from build123d import *

# Parameters (mm, degrees)
BOSS_EXTRUDE1_DEPTH = 5
CIRPATTERN1_COUNT   = 3
CIRPATTERN1_ANGLE   = 120
SKETCH8_R           = 22.5
BOSS_EXTRUDE4_DEPTH = 10
SKETCH11_R          = 22.5
CUT_EXTRUDE4_DEPTH  = 11.7
SKETCH12_R          = 4
CUT_EXTRUDE5_DEPTH  = 3.3
SKETCH14_R          = 3.65
CUT_EXTRUDE7_DEPTH  = 100.784323589
CIRPATTERN2_COUNT   = 6
CUT_EXTRUDE9_DEPTH  = 15


# Read off the part's stored shape, not the designer's step: Boundary2
with BuildPart() as part:
    # Sketch1 → Boss-Extrude1 (new body)
    with BuildSketch(Plane(origin=(0, 0, 0), x_dir=(1, 0, 0), z_dir=(0, 1, 0))):
        with BuildLine():
            ThreePointArc((-15.9, 47.404535648), (-50, 0), (-15.9, -47.404535648))
            Line((-15.9, -47.404535648), (-15.9, 47.404535648))
        make_face()
        with BuildLine():
            ThreePointArc((-15.9, -47.404535648), (0, -50), (15.9, -47.404535648))
            Line((15.9, -47.404535648), (15.9, 47.404535648))
            ThreePointArc((15.9, 47.404535648), (0, 50), (-15.9, 47.404535648))
            Line((-15.9, 47.404535648), (-15.9, -47.404535648))
        make_face()
        with BuildLine():
            Line((-15.9, -70.5), (15.9, -70.5))
            Line((15.9, -70.5), (15.9, -47.404535648))
            ThreePointArc((15.9, -47.404535648), (0, -50), (-15.9, -47.404535648))
            Line((-15.9, -47.404535648), (-15.9, -70.5))
        make_face()
        with BuildLine():
            ThreePointArc((-15.9, 47.404535648), (0, 50), (15.9, 47.404535648))
            Line((15.9, 47.404535648), (15.9, 70.5))
            Line((15.9, 70.5), (-15.9, 70.5))
            Line((-15.9, 70.5), (-15.9, 47.404535648))
        make_face()
        with BuildLine():
            Line((15.9, 47.404535648), (15.9, -47.404535648))
            ThreePointArc((15.9, -47.404535648), (40.589407485, -29.197602641), (50, 0))
            ThreePointArc((50, 0), (40.589407485, 29.197602641), (15.9, 47.404535648))
        make_face()
    boss_extrude1 = extrude(amount=BOSS_EXTRUDE1_DEPTH)

    # CirPattern1: Boss-Extrude1 ×3 about axis
    cirpattern1_axis = Axis((0, 0, 0), (0, 1, 0))
    for i in range(1, CIRPATTERN1_COUNT):
        add(boss_extrude1.rotate(cirpattern1_axis, i * CIRPATTERN1_ANGLE / (CIRPATTERN1_COUNT - 1)))

    # Sketch8 → Boss-Extrude4 (add)
    with BuildSketch(Plane(origin=(0, 5, 0), x_dir=(1, 0, 0), z_dir=(0, 1, 0))):
        with Locations(Location((0, 0, 0), (0, 0, 270))):
            Circle(SKETCH8_R)
    extrude(amount=BOSS_EXTRUDE4_DEPTH)

    # Boundary2 outline → Boundary2 (revolve)
    with BuildSketch(Plane.XY):
        Polygon((32.5, 5), (22.499998072, 15.000001928), (22.5, 5), align=None)
    revolve(axis=Axis((0, 0, 0), (0, 1, 0)))

    # Sketch11 → Cut-Extrude4 (cut)
    with BuildSketch(Plane.XZ):
        with Locations(Location((0, 0, 0), (0, 0, 270))):
            Circle(SKETCH11_R)
    extrude(amount=-CUT_EXTRUDE4_DEPTH, mode=Mode.SUBTRACT)

    # Sketch12 → Cut-Extrude5 (cut)
    with BuildSketch(Plane.XZ.offset(-11.7)):
        with Locations(Location((0, 0, 0), (0, 0, 270))):
            Circle(SKETCH12_R)
    extrude(amount=-CUT_EXTRUDE5_DEPTH, mode=Mode.SUBTRACT)

    # Sketch14 → Cut-Extrude7 (cut, through all)
    with BuildSketch(Plane(origin=(0, 0, 0), x_dir=(-1, 0, 0), z_dir=(0, -1, 0))):
        with Locations(Location((5.17, -60, 0), (0, 0, 90))):
            Circle(SKETCH14_R)
    cut_extrude7 = extrude(amount=-CUT_EXTRUDE7_DEPTH, mode=Mode.SUBTRACT)

    # CirPattern2: Cut-Extrude7 ×6 about axis
    cirpattern2_axis = Axis((0, 0, 0), (0, 1, 0))
    for i in range(1, CIRPATTERN2_COUNT):
        add(cut_extrude7.rotate(cirpattern2_axis, i * 360 / CIRPATTERN2_COUNT), mode=Mode.SUBTRACT)

    # Sketch15 → Cut-Extrude9 (cut)
    with BuildSketch(Plane(origin=(0, 5, 0), x_dir=(1, 0, 0), z_dir=(0, 1, 0))):
        with BuildLine():
            Line((-37.776643972, 13.150101528), (-31.136127875, 9.316197772))
            ThreePointArc((-31.136127875, 9.316197772), (-32.5, 0), (-31.136127875, -9.316197772))
            Line((-31.136127875, -9.316197772), (-37.776643972, -13.150101528))
            ThreePointArc((-37.776643972, -13.150101528), (-40, 0), (-37.776643972, 13.150101528))
        make_face()
        with BuildLine():
            Line((-30.276643972, 26.140482585), (-23.636127875, 22.306578829))
            ThreePointArc((-23.636127875, 22.306578829), (-16.25, 28.145825623), (-7.5, 31.622776602))
            Line((-7.5, 31.622776602), (-7.5, 39.290584114))
            ThreePointArc((-7.5, 39.290584114), (-20, 34.641016151), (-30.276643972, 26.140482585))
        make_face()
        with BuildLine():
            Line((7.5, 39.290584114), (7.5, 31.622776602))
            ThreePointArc((7.5, 31.622776602), (16.25, 28.145825623), (23.636127875, 22.306578829))
            Line((23.636127875, 22.306578829), (30.276643972, 26.140482585))
            ThreePointArc((30.276643972, 26.140482585), (20, 34.641016151), (7.5, 39.290584114))
        make_face()
        with BuildLine():
            Line((37.776643972, 13.150101528), (31.136127875, 9.316197772))
            ThreePointArc((31.136127875, 9.316197772), (32.5, 0), (31.136127875, -9.316197772))
            Line((31.136127875, -9.316197772), (37.776643972, -13.150101528))
            ThreePointArc((37.776643972, -13.150101528), (40, 0), (37.776643972, 13.150101528))
        make_face()
        with BuildLine():
            Line((30.276643972, -26.140482585), (23.636127875, -22.306578829))
            ThreePointArc((23.636127875, -22.306578829), (16.25, -28.145825623), (7.5, -31.622776602))
            Line((7.5, -31.622776602), (7.5, -39.290584114))
            ThreePointArc((7.5, -39.290584114), (20, -34.641016151), (30.276643972, -26.140482585))
        make_face()
        with BuildLine():
            Line((-7.5, -39.290584114), (-7.5, -31.622776602))
            ThreePointArc((-7.5, -31.622776602), (-16.25, -28.145825623), (-23.636127875, -22.306578829))
            Line((-23.636127875, -22.306578829), (-30.276643972, -26.140482585))
            ThreePointArc((-30.276643972, -26.140482585), (-20, -34.641016151), (-7.5, -39.290584114))
        make_face()
    extrude(amount=-CUT_EXTRUDE9_DEPTH, mode=Mode.SUBTRACT)


solid = part.part
Build history of the part. All positions in model axes, mm. A direction names the side the tool comes from. Coordinates: 2 decimals unless noted, no trailing zeros. Write each loop counter-clockwise with the first axis right and the second up, starting at its lowest first coordinate (ties: lowest second). Pieces come first, ordered by that corner, then holes. Notation, with made-up numbers: (-6.75, 34) -> (6.25, 34) arc R30 ccw to (6.25, 58) -> close; hole circle Ø9 at (4.25, 58.5). An arc over 180 degrees is marked (long way). Use CSV: the item, a comma, the result in double quotes. Start each with the question number.
Q1. Pull direction Z, two halves, no side cores. Call faces 1 (the cylindrical face through (-54.707, 2.465, 21.876)), 2 (the flat face through (-5, 15, 0)), 3 (the cylindrical face through (-24.88, 2.46, -43.37)): released by +Z, released by -Z, zero draft, split by the parting line, or undercut.
Q2. 3-axis set-ups, long thin cutter, end or side, ignore diameter. For faces 4 (the flat face through (-42.964, 2.465, -43.165)), 5 (the cylindrical face through (-8.618, 5.768, -20.784)), 6 (the flat face through (-43.2, 2.5, 43.3)), 7 (the flat face through (-59.144, 2.465, -15.787)), 8 (the flat face through (-7.5, 3, 36)): which of +Z, -Z, +X, -X, +Y, -Y reach the whole face in a straight line?
Q3. Cut at A-A, the plane z = -60. List the corners of the cut face in (x, y), then the cut area to 4 significant figures.
Q4. Cut at D-D, the plane y = 8. List the corners of the cut face in (x, z), then the cut area to 3 significant figures.
Q5. Cut at C-C, the plane z = -45. List the corners of the cut face in (x, y).
Q6. Cut at B-B, the plane x = 60.5. List the corners of the cut face in (y, z), then the cut area to 3 significant figures.
Q7. Drill centre lines: probe 1 along X at (y, z) = (1.5, 60); probe 2 along X at (y, z) = (4.75, 7.5); probe 3 along X at (y, z) = (1.25, -43.5). Where is each one in solid material? Low to high.
Q8. Flat gauge pins, fed straight in: pin 1 Ø11.5 at (x, z) = (54.55, -25.52) entering from +Y; pin 2 Ø13.5 at (x, z) = (-7.5, 4) entering from -Y; pin 3 Ø1.5 at (y, z) = (3.5, 60) entering from +X. Where does each tip first touch, or does it go through?
Checked values:
1,face 1,"undercut"
1,face 2,"zero draft"
1,face 3,"released by -Z"
2,face 4,"-Z, +Y, -Y"
2,face 5,"-Y"
2,face 6,"+Z, +Y, -Y"
2,face 7,"-X, +Y, -Y"
2,face 8,"+Y, -Y"
3,outline,"(-15.9, 0) -> (1.52, 0) -> (1.52, 5) -> (-15.9, 5) -> close; (8.82, 0) -> (15.9, 0) -> (15.9, 5) -> (8.82, 5) -> close"
3,area,"122.5 mm²"
4,outline,"circle Ø59 at (0, 0); hole circle Ø45 at (0, 0)"
4,area,"1,140 mm²"
5,outline,"(-55.43, 0) -> (-46.14, 0) -> (-46.14, 5) -> (-55.43, 5) -> close; (-21.79, 0) -> (21.79, 0) -> (21.79, 5) -> (-21.79, 5) -> close; (46.14, 0) -> (55.43, 0) -> (55.43, 5) -> (46.14, 5) -> close"
6,outline,"(0, -36.21) -> (5, -36.21) -> (5, -16.57) -> (0, -16.57) -> close; (0, 16.57) -> (5, 16.57) -> (5, 36.21) -> (0, 36.21) -> close"
6,area,"196 mm²"
7,probe 1,"x = -15.9 to -8.82, -1.52 to 15.9"
7,probe 2,"x = -49.43 to -39.29, -31.62 to -21.21, 21.21 to 31.62, 39.29 to 49.43"
7,probe 3,"x = -56.29 to -43.54, -24.65 to 24.65, 43.54 to 56.29"
8,pin 1,"stops at y = 5"
8,pin 2,"stops at y = 11.7"
8,pin 3,"stops at x = 15.9"
